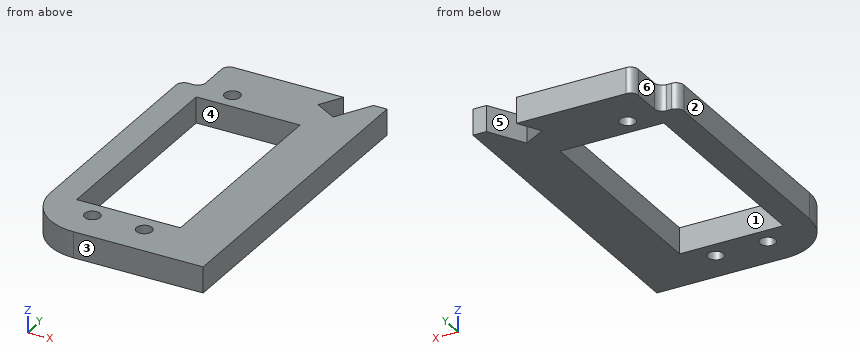
```python
from build123d import *

# Parameters (mm, degrees)
ESQUISSE1_R        = 1.5
BOSS_EXTRU_1_DEPTH = 5
CONG_2_R           = 10
CONG_4_R           = 1.5


with BuildPart() as part:
    # Esquisse1 → Boss.-Extru.1 (new body)
    with BuildSketch(Plane.XY):
        Polygon((0, 0), (25, 0), (35, 0), (35, 63), (32.405486101, 63), (28.462110428, 56.169872981), (24.131983409, 58.669872981), (26.631983409, 63), (4, 63), (4, 54.5), (0, 54.5), align=None)
        with Locations((10, 54.5)):
            Circle(ESQUISSE1_R, mode=Mode.SUBTRACT)
        with Locations((20, 6.5)):
            Circle(ESQUISSE1_R, mode=Mode.SUBTRACT)
        with Locations((10, 6.5)):
            Circle(ESQUISSE1_R, mode=Mode.SUBTRACT)
        Polygon((15, 51), (5, 51), (5, 10), (25, 10), (25, 51), align=None, mode=Mode.SUBTRACT)
    extrude(amount=BOSS_EXTRU_1_DEPTH)

    # Congé2
    cong_2_edges = [part.edges().sort_by_distance(p)[0] for p in [
        (0, 0, 2.5),
    ]]
    fillet(cong_2_edges, radius=CONG_2_R)

    # Congé4
    cong_4_edges = [part.edges().sort_by_distance(p)[0] for p in [
        (0, 54.5, 2.5),
        (4, 54.5, 2.5),
        (4, 63, 2.5),
    ]]
    fillet(cong_4_edges, radius=CONG_4_R)


solid = part.part
```
Here's how the part is built. I have some questions about the finished solid (model axes, mm). Face numbers are marked on the shaded views. A direction names the side the tool comes from. Round coordinates to 2 decimals unless told otherwise and drop trailing zeros. Write each loop counter-clockwise with the first axis right and the second up, starting at its lowest first coordinate (ties: lowest second). Pieces come first, ordered by that corner, then holes.
Q1. Which directions (+Z, -Z, +X, -X, +Y, -Y) give clear straight access to the entire face, cutting with the end or side of a thin tool? Please do the marked faces 4, 5 and 6.
Q2. Please list where these lines run through material, in increasing order: probe 1 along Y at (x, z) = (10, 3.1); probe 2 along Y at (x, z) = (20, 3.75); probe 3 along Y at (x, z) = (18, 0.45).
Q3. If we section it at A-A on x = 23: Write out the boundary of the cut face in (y, z).
Q4. If we section it at B-B on y = 17: Write out the boundary of the cut face in (x, z).
Q5. If we section it at D-D on y = 6.5: Write out the boundary of the cut face in (x, z), plus the area to 3 significant figures.
Q6. If we section it at C-C on z = 0.9: Write out the boundary of the cut face in (x, y), plus the area to 3 significant figures.
Q7. Will these pins go through, and if not, where does the flat tip stop? P1, Ø3, axis at x = 7, y = 40, coming from the -Z side; P2, Ø1.1, axis at x = 2, z = 2.5, coming from the +Y side; P3, Ø2.5, axis at y = 57.5, z = 2.5, coming from the -X side.
Q8. If we mould it in two halves opening along Y, with no side actions, what happens to the marked faces 1, 2 and 3? For each: +Y half, -Y half, draft (parallel to the pull), parting line (faces both ways), or undercut.
Answer below:
1. face 4: +Z, -Z
1. face 5: +Z, -Z, +Y
1. face 6: +Z, -Z, -X, +Y
2. probe 1: y = 0 to 5, 8 to 10, 51 to 53, 56 to 63
2. probe 2: y = 0 to 5, 8 to 10, 51 to 63
2. probe 3: y = 0 to 10, 51 to 63
3. outline: (0, 0) - (10, 0) - (10, 5) - (0, 5) - close; (51, 0) - (63, 0) - (63, 5) - (51, 5) - close
4. outline: (0, 0) - (5, 0) - (5, 5) - (0, 5) - close; (25, 0) - (35, 0) - (35, 5) - (25, 5) - close
5. outline: (0.63, 0) - (8.5, 0) - (8.5, 5) - (0.63, 5) - close; (11.5, 0) - (18.5, 0) - (18.5, 5) - (11.5, 5) - close; (21.5, 0) - (35, 0) - (35, 5) - (21.5, 5) - close
5. area: 142 mm2
6. outline: (0, 10) arc R10 ccw to (10, 0) - (35, 0) - (35, 63) - (32.41, 63) - (28.46, 56.17) - (24.13, 58.67) - (26.63, 63) - (5.5, 63) arc R1.5 ccw to (4, 61.5) - (4, 56) arc R1.5 cw to (2.5, 54.5) - (1.5, 54.5) arc R1.5 ccw to (0, 53) - close; hole (5, 10) - (25, 10) - (25, 51) - (5, 51) - close; hole circle Ø3 at (10, 6.5); hole circle Ø3 at (10, 54.5); hole circle Ø3 at (20, 6.5)
6. area: 1,280 mm2
7. P1: passes through
7. P2: stops at y = 54.5
7. P3: stops at x = 4
8. face 1: undercut
8. face 2: draft
8. face 3: -Y half
